Input: part model. Units: mm. Frame: model coordinates. A direction names the side the tool comes from. Round coordinates to 2 decimals unless told otherwise and drop trailing zeros. Loops run counter-clockwise (first coordinate to the right, second up) from the corner with the lowest first, then second, coordinate; pieces in that order, holes last. Notation, with made-up numbers: (8, 49) -> (66, 49) arc R20 ccw to (66, 84) -> close; hole circle Ø5 at (12, 45). An arc over 180 degrees is marked (long way). Answer as a JSON object with one key per item and string values. Group by question number.
Item 1: Set-up query: faces 5 (the flat face through (1, 1, 27.4)), 6 (the flat face through (-37, 1, -13.5)), 7 (the flat face through (34.9, 1, -6)). Return all of +Z, -Z, +X, -X, +Y, -Y with unobstructed straight access to the full face (end or side cutting, diameter ignored); none if empty.
Item 2: Material intervals for line 1 (X direction, y = 0.45, z = 14.45); line 2 (Z direction, x = 37.15, y = 0.7); line 3 (X direction, y = 1.4, z = -21.5), sorted ascending. Write a range as [from, to].
Item 3: Pin query (flat end, axial travel): pin 1 (3 mm diameter, centred on x = 37.15, z = 14.45, fed in from +Y); pin 2 (1.4 mm diameter, centred on x = 37.15, z = -20.45, fed in from -Y); pin 3 (0.5 mm diameter, centred on y = 1, z = -7, fed in from -X). Return the tip coordinate at first contact, or that it passes through.
Item 4: Section query B-B on x = -37.15. Return loops of the section in (y, z).
Item 5: Section query C-C on y = 0.7. Return loops of the section in (x, z), and give its area (3 significant figures).
Item 6: Section query A-A on z = -20.45. Return loops of the section in (x, y), and give its area (3 significant figures).
Item 7: Draft query along Z for faces 1 (the flat face through (-34.9, 1, -6)), 2 (the flat face through (39.4, 1, -20)), 3 (the cylindrical face through (-35.98, 0.79, 14.19)), 4 (the flat face through (-1, 1, -27.4)). Return one class per face: released by +Z, released by -Z, zero draft, split by the parting line, or undercut.
Autodesk Inventor part; units mm, degrees
ref_plane "YZ Plane" through (0, 0, 0) normal (1, 0, 0) x (0, 1, 0)
ref_plane "XZ Plane" through (0, 0, 0) normal (0, 1, 0) x (-1, 0, 0)
ref_plane "XY Plane" through (0, 0, 0) normal (0, 0, 1) x (1, 0, 0)
sketch "スケッチ1" plane through (0, 0, 0) normal (0, 1, 0) x (-1, 0, 0)
  line L0 (39.4, -27.4) -> (0, -27.4)
  line L1 (0, -27.4) -> (0, 27.4)
  line L2 (0, 27.4) -> (39.4, 27.4)
  line L3 (39.4, -13.5) -> (34.9, -13.5)
  line L4 (34.9, -13.5) -> (34.9, 1.5)
  line L5 (34.9, 1.5) -> (39.4, 1.5)
  line L6 (39.4, 1.5) -> (39.4, -13.5) construction
  line L7 (39.4, 27.4) -> (39.4, 1.5)
  line L8 (39.4, -13.5) -> (39.4, -27.4)
  line L9 (0, -22.4) -> (15, -22.4)
  line L10 (15, -22.4) -> (15, -2.4)
  line L11 (15, -2.4) -> (0, -2.4)
  line L12 (-39.4, -27.4) -> (0, -27.4)
  line L13 (0, 27.4) -> (-39.4, 27.4)
  line L14 (-39.4, -13.5) -> (-34.9, -13.5)
  line L15 (-34.9, -13.5) -> (-34.9, 1.5)
  line L16 (-34.9, 1.5) -> (-39.4, 1.5)
  line L17 (-39.4, 1.5) -> (-39.4, -13.5) construction
  line L18 (-39.4, 27.4) -> (-39.4, 1.5)
  line L19 (-39.4, -13.5) -> (-39.4, -27.4)
  line L20 (0, -22.4) -> (-15, -22.4)
  line L21 (-15, -22.4) -> (-15, -2.4)
  line L22 (-15, -2.4) -> (0, -2.4)
  point P0 (0, 0)
  point P1 (0, 0)
  point P2 (0, 0)
  dimension "d0" = 13.9
  dimension "d1" = 25.9
  dimension "d2" = 39.4
  dimension "d3" = 15
  dimension "d4" = 4.5
  dimension "d5" = 20
  dimension "d6" = 15
  dimension "d7" = 5
extrude "押し出し1" add sketch "スケッチ1" along normal blind 1.6 contours L0 L1 L9 L10 L11 L2 L7 L5 L4 L3 L8 | L12 L19 L14 L15 L16 L18 L13 L1 L22 L21 L20
sketch "スケッチ2" plane through (0, 1.6, 0) normal (0, 1, 0) x (1, 0, 0)
  line L0 (-39.4, 13.5) -> (-34.9, 13.5)
  line L1 (-37.15, 13.5) -> (-37.15, 27.4) construction
  line L2 (-34.9, -1.5) -> (-39.4, -1.5)
  line L3 (-37.15, -1.5) -> (-37.15, -27.4) construction
  line L4 (-39.4, -27.4) -> (39.4, -27.4)
  line L5 (39.4, 27.4) -> (-39.4, 27.4)
  point P0 (0, 0)
  point P1 (-37.15, 20.45)
  point P2 (-37.15, -14.45)
hole "穴1" at (-37.15, 1.6, -20.45) at (-37.15, 1.6, 14.45) direction (0, -1, 0) diameter 2.4 end through all
ref_plane "作業平面1" through (0, 0, -13.5) normal (-1, 0, 0) x (0, 0, 1)
mirror "ミラー1" about plane through (0, 0, -13.5) normal (-1, 0, 0) of "穴1"
sketch "スケッチ3" plane through (0, 1.6, 0) normal (0, 1, 0) x (1, 0, 0)
  line L0 (15, 22.4) -> (15, 2.4)
  line L1 (-15, 22.4) -> (15, 22.4)
  line L2 (15, 22.4) -> (15, 2.4)
  line L3 (15, 2.4) -> (-15, 2.4)
  line L4 (-15, 2.4) -> (-15, 22.4)
  point P0 (0, 0)
extrude "押し出し2" add sketch "スケッチ3" against normal up to surface (1.6 mm away)
properties part number "top" material "エポキシ樹脂"
Solved:
{
 "1": {"face 5": "+Z, +X, -X, +Y, -Y", "face 6": "-X, +Y, -Y", "face 7": "+X, +Y, -Y"},
 "2": {"line 1": "[-39.4, -38.35], [-35.95, 35.95], [38.35, 39.4]", "line 2": "[-27.4, -21.65], [-19.25, -13.5], [1.5, 13.25], [15.65, 27.4]", "line 3": "[-39.4, -37.73], [-36.57, 36.57], [37.73, 39.4]"},
 "3": {"pin 1": "y = 1.6", "pin 2": "through", "pin 3": "x = -34.9"},
 "4": {"outline": "(0, -27.4) -> (1.6, -27.4) -> (1.6, -21.65) -> (0, -21.65) -> close; (0, -19.25) -> (1.6, -19.25) -> (1.6, -13.5) -> (0, -13.5) -> close; (0, 1.5) -> (1.6, 1.5) -> (1.6, 13.25) -> (0, 13.25) -> close; (0, 15.65) -> (1.6, 15.65) -> (1.6, 27.4) -> (0, 27.4) -> close"},
 "5": {"outline": "(-39.4, -27.4) -> (39.4, -27.4) -> (39.4, -13.5) -> (34.9, -13.5) -> (34.9, 1.5) -> (39.4, 1.5) -> (39.4, 27.4) -> (-39.4, 27.4) -> (-39.4, 1.5) -> (-34.9, 1.5) -> (-34.9, -13.5) -> (-39.4, -13.5) -> close; hole circle Ø2.4 at (-37.15, -20.45); hole circle Ø2.4 at (-37.15, 14.45); hole circle Ø2.4 at (37.15, -20.45); hole circle Ø2.4 at (37.15, 14.45)", "area": "4,170 mm²"},
 "6": {"outline": "(-39.4, 0) -> (-38.35, 0) -> (-38.35, 1.6) -> (-39.4, 1.6) -> close; (-35.95, 0) -> (35.95, 0) -> (35.95, 1.6) -> (-35.95, 1.6) -> close; (38.35, 0) -> (39.4, 0) -> (39.4, 1.6) -> (38.35, 1.6) -> close", "area": "118 mm²"},
 "7": {"face 1": "undercut", "face 2": "zero draft", "face 3": "undercut", "face 4": "released by -Z"}
}
